Geometry check sheet. Reference: the model listing, model coordinates, mm. A direction names the side the tool comes from. Give positions to 0.01 mm unless a question says otherwise; leave off trailing zeros. Write each loop counter-clockwise with the first axis right and the second up, starting at its lowest first coordinate (ties: lowest second). Pieces come first, ordered by that corner, then holes. Notation, with made-up numbers: (30.25, 13) - (42.25, 13) arc R15 ccw to (42.25, 29) - close; hole circle Ø1 at (88.25, 63). An arc over 180 degrees is marked (long way). One line per question, with ' | ' between items. Start each with the question number.
Q1. Gauge pin test, flat ends, axial feed: P1, Ø1.5, axis at x = -47, z = 119, coming from the +Y side; P2, Ø10, axis at y = 55, z = -30, coming from the +X side; P3, Ø8, axis at x = -135.5, y = -80.5, coming from the -Z side. Record the tip position at first contact, or that the pin passes through.
Q2. Section check A-A on z = 152.4. Record the boundary of the cut face in (x, y).
Q3. Section check D-D on x = -34. Record the boundary of the cut face in (y, z).
Q4. Set-up check for faces 4 (the face through (-75.639, -60.47, 46.367)), 5 (the face through (-99.62, -114.19, -5.03)), 6 (the face through (-36.65, -144.771, -24.227)): record each of +Z, -Z, +X, -X, +Y, -Y from which the full face is reachable in a straight line by a thin tool's end or side.
Q5. Release check for a two-part mould opening along Y. For faces 1 (the face through (-24.128, 87, -3)), 2 (the face through (-36.65, -44.05, 198.368)), 3 (the face through (-36.65, 127.604, 5.506)) record: +Y half, -Y half, draft (parallel to the pull), parting line (faces both ways), or undercut.
Q6. Thickness scan on L1, parallel to Y at x = -36.75, z = 0; L2, parallel to Y at x = -42, z = 6.5; L3, parallel to Y at x = -100, z = 0. Record the ranges inside material, lowest first. Write a range as [from, to].
Q7. Section check B-B on y = 0. Record the boundary of the cut face in (x, z).
```python
from build123d import *

# Parameters (mm, degrees)
SKETCH2_R          = 25.4
CUT_EXTRUDE1_DEPTH = 128


with BuildPart() as part:
    # Sketch1 → Revolve1 (revolve)
    with BuildSketch(Plane.XY):
        Polygon((-151.127552987, 114.3), (-49.527552987, 114.3), (-49.527552987, 203.2), (-24.127552987, 203.2), (-24.127552987, 76.2), (-125.727552987, 76.2), (-125.727552987, 50.8), (-151.127552987, 50.8), align=None)
    revolve(axis=Axis((0, 0, 0), (-1, 0, 0)))

    # Sketch2 → Cut-Extrude1 (cut, through all)
    with BuildSketch(Plane(origin=(-24.127552987, 0, 0), x_dir=(0, 0, -1), z_dir=(1, 0, 0))):
        with Locations((0, 152.4)):
            Circle(SKETCH2_R)
        with Locations((-152.4, 0)):
            Circle(SKETCH2_R)
        with Locations((152.4, 0)):
            Circle(SKETCH2_R)
        with Locations((0, -152.4)):
            Circle(SKETCH2_R)
    extrude(amount=-CUT_EXTRUDE1_DEPTH, mode=Mode.SUBTRACT)


solid = part.part
```
Working result:
1) P1: stops at y = 165.25 | P2: stops at x = -125.73 | P3: stops at z = -84.92
2) outline: (-49.53, -134.4) - (-24.13, -134.4) - (-24.13, -25.4) - (-49.53, -25.4) - close; (-49.53, 25.4) - (-24.13, 25.4) - (-24.13, 134.4) - (-49.53, 134.4) - close
3) outline: circle Ø406.4 at (0, 0); hole circle Ø50.8 at (-152.4, 0); hole circle Ø152.4 at (0, 0); hole circle Ø50.8 at (0, -152.4); hole circle Ø50.8 at (0, 152.4); hole circle Ø50.8 at (152.4, 0)
4) face 4: +X | face 5: -X | face 6: +X, -X
5) face 1: draft | face 2: parting line | face 3: undercut
6) L1: y = [-203.2, -177.8], [-127, -76.2], [76.2, 127], [177.8, 203.2] | L2: y = [-203.1, -176.95], [-127.85, -75.92], [75.92, 127.85], [176.95, 203.1] | L3: y = [-114.3, -76.2], [76.2, 114.3]
7) outline: (-151.13, -114.3) - (-49.53, -114.3) - (-49.53, -127) - (-24.13, -127) - (-24.13, -76.2) - (-125.73, -76.2) - (-125.73, -50.8) - (-151.13, -50.8) - close; (-151.13, 50.8) - (-125.73, 50.8) - (-125.73, 76.2) - (-24.13, 76.2) - (-24.13, 127) - (-49.53, 127) - (-49.53, 114.3) - (-151.13, 114.3) - close; (-49.53, -203.2) - (-24.13, -203.2) - (-24.13, -177.8) - (-49.53, -177.8) - close; (-49.53, 177.8) - (-24.13, 177.8) - (-24.13, 203.2) - (-49.53, 203.2) - close
